Can you work these out from the model? Positions are in its coordinate system, mm. A direction names the side the tool comes from. Give positions to 0.01 mm unless a question says otherwise; leave off trailing zeros. Loops run counter-clockwise (first coordinate to the right, second up) from the corner with the lowest first, then second, coordinate; pieces in that order, holes last. Notation, with made-up numbers: (87, -28) -> (144, -28) arc R19 ccw to (144, 1) -> close; hole circle Ø3 at (49, 88.25). An arc over 180 degrees is marked (long way). Return JSON: item names as keys, results as strings. Group by question number.
Q1. Suppose I cut it at D-D, the plane x = 2.25. Please give me the cut outline in (y, z), and give its area (3 significant figures).
Q2. Will these pins go through, and if not, where does the flat tip stop? pin 1 (3 mm diameter, centred on x = 3, y = 4.5, fed in from +Z); pin 2 (2 mm diameter, centred on x = 1.5, y = 1.5, fed in from +Z); pin 3 (4 mm diameter, centred on x = 4, y = -4, fed in from +Z); pin 4 (5 mm diameter, centred on x = -1.5, z = -1, fed in from +Y).
Q3. I need wall thicknesses on line 1 along X through (y, z) = (3.5, 3.25); line 2 along Z through (x, y) = (1, 0.75); line 3 along X through (y, z) = (-3.25, -4). Which ranges of each line are inside material? Lowest first, please. Write a range as [from, to].
Q4. Which directions (+Z, -Z, +X, -X, +Y, -Y) give clear straight access to the entire face, cutting with the end or side of a thin tool? Please do faces 1 (the cylindrical face through (-2.058, 2.681, 6.466)), 2 (the cylindrical face through (2.18, 1.08, -4.88)).
Q5. Suppose I cut it at C-C, the plane x = -1.5. Please give me the cut outline in (y, z).
```python
from build123d import *

# Parameters (mm, degrees)
F2_R     = 5
F3_DEPTH = 8
F4_R     = 4.5
F5_DEPTH = 1
F6_SIZE  = 0.99999


# Not quite as in the source:
# - a fillet or chamfer is up to 0.001 mm smaller than in the source, because OpenCascade refuses the exact size


with BuildPart() as f1:
    # F0 (on Front) → F1 (revolve)
    with BuildSketch(Plane.XZ):
        with BuildLine():
            Line((-3.0435194335, 0), (0, 0))
            ThreePointArc((0, 0), (-0.2623133647, 3.5386767586), (-1.0435194335, 7))
            Line((-1.0435194335, 7), (-3.0435194335, 7))
            Line((-3.0435194335, 7), (-3.0435194335, 0))
        make_face()
    revolve(axis=Axis((-1.5217597168, 0, 0), (1, 0, 0)))

    # F2 (on face) → F3 (join)
    with BuildSketch(Plane(origin=(-3.0435194335, 0, 0), x_dir=(0, -1, 0), z_dir=(-1, 0, 0))):
        Circle(F2_R)
    extrude(amount=-F3_DEPTH)

    # F4 (on face) → F5 (join)
    with BuildSketch(Plane.YZ.offset(4.9564805665)):
        Circle(F4_R)
    extrude(amount=F5_DEPTH)

    # F6 (size 1 in the source; OpenCascade refuses exactly that, so slightly less here)
    f6_edges = [f1.edges().sort_by_distance(p)[0] for p in [
        (5.956481, -4.5, 0),
    ]]
    chamfer(f6_edges, length=F6_SIZE)


solid = f1.part
```
Ans:
{
 "1": {"outline": "circle Ø10 at (0, 0)", "area": "78.5 mm^2"},
 "2": {"pin 1": "stops at z = 4", "pin 2": "stops at z = 4.97", "pin 3": "stops at z = 4.58", "pin 4": "stops at y = 7"},
 "3": {"line 1": "x = [-3.04, 4.96]", "line 2": "z = [-4.94, 4.94]", "line 3": "x = [-3.04, -0.56]"},
 "4": {"face 1": "+X, -X", "face 2": "+X"},
 "5": {"outline": "circle Ø14 at (0, 0)"}
}
